The drawing under review shows one solid part. Ordinate dimensions are in mm from its lowest x, y, z. Give positions to 0.01 mm unless a question says otherwise; leave off trailing zeros. Write each loop counter-clockwise with the first axis right and the second up, starting at its lowest first coordinate (ties: lowest second). Pieces come first, ordered by that corner, then holes. Notation, with made-up numbers: M -21.5,87.5 L 14.5,87.5 A11 cw 14.5,104.5 Z; hole C 82,64.5 d2. An arc over 180 degrees is marked long. Use one line per item in the form item = value. Start each with the question number.
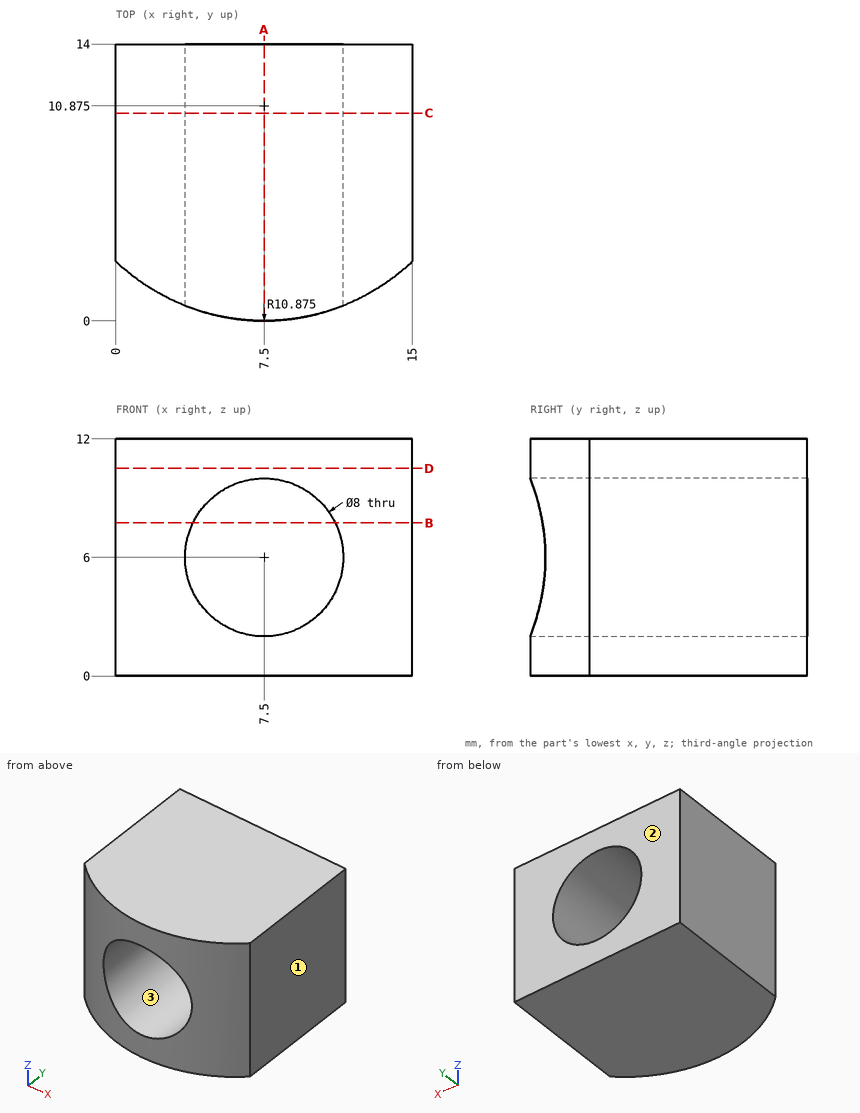
1. We need section D-D (z = 10.5). State the section outline as (x, y) points (3 decimals), and give its area (3 significant figures).
2. Draft analysis for pull direction X (two halves, no side actions). For the marked faces 1, 2 and 3, state which applies: pulls with the +X half, pulls with the -X half, needs draft (parallel to the pull), parting line crosses it, or undercut.
3. We need section C-C (y = 10.5). State the section outline as (x, z) points, and give its area (3 significant figures).
4. To check wall thickness, follow L1, parallel to X at y = 9, z = 6; L2, parallel to Z at x = 7.25, y = 8.75; L3, parallel to Z at x = 4.5, y = 4.5. State the ranges of each line that lie inside material, in increasing order.
5. We need section A-A (x = 7.5). State the section outline as (y, z) points, and give its area (3 significant figures).
6. We need section B-B (z = 7.75). State the section outline as (x, y) points (3 decimals), and give its area (3 significant figures).
7. Clearance check with a flat-ended pin moving along its axis: pin 1 Ø6 at (x, z) = (2, 2) entering from -Y. State where the tip first meets the part, or that it passes through.
Answer block:
q1.outline = M 0,3 A10.875 ccw 15,3 L 15,14 L 0,14 Z
q1.area = 196 mm^2
q2.face_1 = pulls with the +X half
q2.face_2 = needs draft
q2.face_3 = undercut
q3.outline = M 0,0 L 15,0 L 15,12 L 0,12 Z; hole C 7.5,6 d8
q3.area = 130 mm^2
q4.L1 = 0 to 3.5, 11.5 to 15
q4.L2 = 0 to 2.01, 9.99 to 12
q4.L3 = 0 to 3.35, 8.65 to 12
q5.outline = M 0,0 L 14,0 L 14,2 L 0,2 Z; M 0,10 L 14,10 L 14,12 L 0,12 Z
q5.area = 56.0 mm^2
q6.outline = M 0,3 A10.875 ccw 3.903,0.612 L 3.903,14 L 0,14 Z; M 11.097,0.612 A10.875 ccw 15,3 L 15,14 L 11.097,14 Z
q6.area = 96.7 mm^2
q7.pin_1 = 0.29
